```python
from build123d import *

# Parameters (mm, degrees)
ESBO_O1_W                                            = 85
ESBO_O1_H                                            = 85
RESSALTO_EXTRUS_O1_DEPTH                             = 8
REBAIXO_PARA_PARAFUSO_DE_M_QUINA_COM_CAB_D           = 4.5
REBAIXO_PARA_PARAFUSO_DE_M_QUINA_COM_CAB_CBORE_D     = 9
REBAIXO_PARA_PARAFUSO_DE_M_QUINA_COM_CAB_CBORE_DEPTH = 3.1
ESBO_O5_W                                            = 30
ESBO_O5_H                                            = 30
RESSALTO_EXTRUS_O2_DEPTH                             = 20
ESBO_O6_R                                            = 10
CORTE_EXTRUS_O1_DEPTH                                = 10
ESBO_O7_R                                            = 10
CORTE_EXTRUS_O2_DEPTH                                = 10
CORTE_EXTRUS_O3_DEPTH                                = 58.5
ESBO_O9_W                                            = 9
ESBO_O9_H                                            = 15
RESSALTO_EXTRUS_O3_DEPTH                             = 10
ESBO_O10_R                                           = 9.75
RESSALTO_EXTRUS_O4_DEPTH                             = 9
ESBO_O11_R                                           = 2
CORTE_EXTRUS_O4_DEPTH                                = 48


with BuildPart() as part:
    # Esboço1 → Ressalto-extrusão1 (new body)
    with BuildSketch(Plane.XY):
        Rectangle(ESBO_O1_W, ESBO_O1_H)
    extrude(amount=RESSALTO_EXTRUS_O1_DEPTH)

    # Rebaixo para parafuso de máquina com cabeça panela de M41 (through all)
    with Locations(Plane.XY.offset(8)):
        with Locations((-36.25, 36.25), (-36.25, -36.25), (36.25, -36.25), (36.25, 36.25)):
            CounterBoreHole(REBAIXO_PARA_PARAFUSO_DE_M_QUINA_COM_CAB_D / 2, REBAIXO_PARA_PARAFUSO_DE_M_QUINA_COM_CAB_CBORE_D / 2, REBAIXO_PARA_PARAFUSO_DE_M_QUINA_COM_CAB_CBORE_DEPTH)

    # Esboço5 → Ressalto-extrusão2 (add)
    with BuildSketch(Plane.XY.offset(8)):
        Rectangle(ESBO_O5_W, ESBO_O5_H)
    extrude(amount=RESSALTO_EXTRUS_O2_DEPTH)

    # Esboço6 → Corte-extrusão1 (cut)
    with BuildSketch(Plane(origin=(15, 0, 0), x_dir=(0, 0, -1), z_dir=(1, 0, 0))):
        with Locations((-28, 0)):
            Circle(ESBO_O6_R)
    extrude(amount=-CORTE_EXTRUS_O1_DEPTH, mode=Mode.SUBTRACT)

    # Esboço7 → Corte-extrusão2 (cut)
    with BuildSketch(Plane.ZY.offset(15)):
        with Locations((28, 0)):
            Circle(ESBO_O7_R)
    extrude(amount=-CORTE_EXTRUS_O2_DEPTH, mode=Mode.SUBTRACT)

    # Esboço8 → Corte-extrusão3 (cut, through all)
    with BuildSketch(Plane.ZY.offset(15)):
        Polygon((18, 10), (18, 15), (28, 15), (28, 10), (28, -10), (28, -15), (18, -15), (18, -10), align=None)
    extrude(amount=-CORTE_EXTRUS_O3_DEPTH, mode=Mode.SUBTRACT)

    # Esboço9 → Ressalto-extrusão3 (add)
    with BuildSketch(Plane.XY.offset(18)):
        Rectangle(ESBO_O9_W, ESBO_O9_H)
    extrude(amount=RESSALTO_EXTRUS_O3_DEPTH)

    # Esboço10 → Ressalto-extrusão4 (add)
    with BuildSketch(Plane.ZY.offset(4.5)):
        with Locations((28, 0)):
            Circle(ESBO_O10_R)
    extrude(amount=-RESSALTO_EXTRUS_O4_DEPTH)

    # Esboço11 → Corte-extrusão4 (cut, through all)
    with BuildSketch(Plane.ZY.offset(4.5)):
        with Locations((28, 0)):
            Circle(ESBO_O11_R)
    extrude(amount=-CORTE_EXTRUS_O4_DEPTH, mode=Mode.SUBTRACT)


solid = part.part
```
Geometry check sheet. Reference: the model listing, model coordinates, mm. A direction names the side the tool comes from. Coordinates: 2 decimals unless noted, no trailing zeros. Loops run counter-clockwise (first coordinate to the right, second up) from the corner with the lowest first, then second, coordinate; pieces in that order, holes last. Notation, with made-up numbers: (76, 11) - (85, 11) arc R31 ccw to (85, 49) - close; hole circle Ø8 at (23, -25.75). An arc over 180 degrees is marked (long way). One line per item, written item: value. Start each with the question number.
(1) Cross-section at C-C on z = 6.5. Enter the section's corners in (x, y).
(2) Tool access check on faces 5 (the cylindrical face through (38.33, 32.26, 6.47)), 6 (the flat face through (-4.5, 0.1, 25.5)), 7 (the flat face through (0, 7.5, 20)). Record the directions out of +Z, -Z, +X, -X, +Y, -Y that give a thin tool (end or side, any length) a straight path to the whole face; none if there is none.
(3) Cross-section at B-B on y = 0. Enter the section's corners in (x, z).
(4) Depth check by flat-ended pin: P1, Ø1, axis at x = -29, z = 9.5, coming from the +Y side; P2, Ø10, axis at x = 34.5, y = -37, coming from the +Z side; P3, Ø2.5, axis at x = -38.5, y = 37.5, coming from the +Z side; P4, Ø2, axis at y = -4.5, z = 23.5, coming from the -X side. Enter the tip coordinate at first touch or a pass-through.
(5) Mould release check, pull along Y, two halves, no side actions. Record for faces 1 (the cylindrical face through (-34.17, -40.24, 6.47)), 2 (the flat face through (-1, 42.5, 4)), 3 (the flat face through (-42.5, -1, 4)), 4 (the flat face through (-34, 34, 4.9)): released by +Y, released by -Y, zero draft, split by the parting line, or undercut.
(6) Cross-section at D-D on x = -36.25. Enter the section's corners in (y, z).
(7) Cross-section at A-A on z = 28. Enter the section's corners in (x, y), plus the area to 4 significant figures.
(8) Material ranges on line 1 (Y direction, x = 36, z = 6); line 2 (Y direction, x = 36, z = 1), recorded low to high. Write a range as [from, to].
Results below:
1. outline: (-42.5, -42.5) - (42.5, -42.5) - (42.5, 42.5) - (-42.5, 42.5) - close; hole circle Ø9 at (-36.25, -36.25); hole circle Ø9 at (-36.25, 36.25); hole circle Ø9 at (36.25, -36.25); hole circle Ø9 at (36.25, 36.25)
2. face 5: +Z
2. face 6: +Z, -X, +Y, -Y
2. face 7: +X, -X, +Y
3. outline: (-42.5, 0) - (42.5, 0) - (42.5, 8) - (15, 8) - (15, 18) - (4.5, 18) - (4.5, 26) - (-4.5, 26) - (-4.5, 18) - (-15, 18) - (-15, 8) - (-42.5, 8) - close; (-4.5, 30) - (4.5, 30) - (4.5, 37.75) - (-4.5, 37.75) - close
4. P1: passes through
4. P2: stops at z = 8
4. P3: stops at z = 4.9
4. P4: stops at x = -4.5
5. face 1: undercut
5. face 2: released by +Y
5. face 3: zero draft
5. face 4: undercut
6. outline: (-42.5, 0) - (-38.5, 0) - (-38.5, 4.9) - (-40.75, 4.9) - (-40.75, 8) - (-42.5, 8) - close; (-34, 0) - (34, 0) - (34, 4.9) - (31.75, 4.9) - (31.75, 8) - (-31.75, 8) - (-31.75, 4.9) - (-34, 4.9) - close; (38.5, 0) - (42.5, 0) - (42.5, 8) - (40.75, 8) - (40.75, 4.9) - (38.5, 4.9) - close
7. outline: (-4.5, -9.75) - (4.5, -9.75) - (4.5, -2) - (-4.5, -2) - close; (-4.5, 2) - (4.5, 2) - (4.5, 9.75) - (-4.5, 9.75) - close
7. area: 139.5 mm2
8. line 1: y = [-42.5, -40.74], [-31.76, 31.76], [40.74, 42.5]
8. line 2: y = [-42.5, -38.49], [-34.01, 34.01], [38.49, 42.5]
